from build123d import *

# Parameters (mm, degrees)
BOSS_EXTRUDE1_DEPTH = 5
SKETCH2_R           = 11.5
BOSS_EXTRUDE2_DEPTH = 35
BOSS_EXTRUDE3_DEPTH = 5
SKETCH4_R           = 0.75
CUT_EXTRUDE1_DEPTH  = 3
CUT_EXTRUDE2_REACH  = 47.957
SKETCH5_R           = 1
CHAMFER1_SIZE       = 1
CUT_EXTRUDE3_REACH  = 52.369
SKETCH6_R           = 8
FILLET2_R           = 5


with BuildPart() as part:
    # Sketch1 → Boss-Extrude1 (new body)
    with BuildSketch(Plane(origin=(0, 0, 0), x_dir=(1, 0, 0), z_dir=(0, 1, 0))):
        with BuildLine():
            Line((-14, 16), (14, 16))
            ThreePointArc((14, 16), (15.414213562, 15.414213562), (16, 14))
            Line((16, 14), (16, -14))
            ThreePointArc((16, -14), (15.414213562, -15.414213562), (14, -16))
            Line((14, -16), (-14, -16))
            ThreePointArc((-14, -16), (-15.414213562, -15.414213562), (-16, -14))
            Line((-16, -14), (-16, 14))
            ThreePointArc((-16, 14), (-15.414213562, 15.414213562), (-14, 16))
        make_face()
    extrude(amount=BOSS_EXTRUDE1_DEPTH)

    # Sketch2 → Boss-Extrude2 (add)
    with BuildSketch(Plane(origin=(0, 5, 0), x_dir=(1, 0, 0), z_dir=(0, 1, 0))):
        with Locations(Location((0, 0, 0), (0, 0, 270))):
            Circle(SKETCH2_R)
    extrude(amount=BOSS_EXTRUDE2_DEPTH)

    # Sketch3 → Boss-Extrude3 (add)
    with BuildSketch(Plane(origin=(0, 40, 0), x_dir=(1, 0, 0), z_dir=(0, 1, 0))):
        with BuildLine():
            Line((-14, 16), (14, 16))
            ThreePointArc((14, 16), (15.414213562, 15.414213562), (16, 14))
            Line((16, 14), (16, -14))
            ThreePointArc((16, -14), (15.414213562, -15.414213562), (14, -16))
            Line((14, -16), (-14, -16))
            ThreePointArc((-14, -16), (-15.414213562, -15.414213562), (-16, -14))
            Line((-16, -14), (-16, 14))
            ThreePointArc((-16, 14), (-15.414213562, 15.414213562), (-14, 16))
        make_face()
    extrude(amount=BOSS_EXTRUDE3_DEPTH)

    # Sketch4 → Cut-Extrude1 (cut)
    with BuildSketch(Plane.XZ):
        with Locations(Location((-13.651323601, 13.573265233, 0), (0, 0, 270))):
            Circle(SKETCH4_R)
        with Locations(Location((13.348541156, 13.658723546, 0), (0, 0, 270))):
            Circle(SKETCH4_R)
        with Locations(Location((13.43399947, -13.34114121, 0), (0, 0, 270))):
            Circle(SKETCH4_R)
        with Locations(Location((-13.565865287, -13.426599524, 0), (0, 0, 270))):
            Circle(SKETCH4_R)
    extrude(amount=-CUT_EXTRUDE1_DEPTH, mode=Mode.SUBTRACT)

    # Sketch5 → Cut-Extrude2 (cut, up to next)
    with BuildSketch(Plane.XZ.offset(-40), mode=Mode.PRIVATE) as cut_extrude2_sk1:
        with Locations(Location((-13.651323601, 13.573265233, 0), (0, 0, 270))):
            Circle(SKETCH5_R)
    cut_extrude2_tool1 = extrude(cut_extrude2_sk1.sketch, amount=-CUT_EXTRUDE2_REACH, mode=Mode.PRIVATE) & part.part
    # Sketch5 → Cut-Extrude2 (cut, up to next)
    with BuildSketch(Plane.XZ.offset(-40), mode=Mode.PRIVATE) as cut_extrude2_sk2:
        with Locations(Location((13.348541156, 13.658723546, 0), (0, 0, 270))):
            Circle(SKETCH5_R)
    cut_extrude2_tool2 = extrude(cut_extrude2_sk2.sketch, amount=-CUT_EXTRUDE2_REACH, mode=Mode.PRIVATE) & part.part
    # Sketch5 → Cut-Extrude2 (cut, up to next)
    with BuildSketch(Plane.XZ.offset(-40), mode=Mode.PRIVATE) as cut_extrude2_sk3:
        with Locations(Location((-13.565865287, -13.426599524, 0), (0, 0, 270))):
            Circle(SKETCH5_R)
    cut_extrude2_tool3 = extrude(cut_extrude2_sk3.sketch, amount=-CUT_EXTRUDE2_REACH, mode=Mode.PRIVATE) & part.part
    # Sketch5 → Cut-Extrude2 (cut, up to next)
    with BuildSketch(Plane.XZ.offset(-40), mode=Mode.PRIVATE) as cut_extrude2_sk4:
        with Locations(Location((13.43399947, -13.34114121, 0), (0, 0, 270))):
            Circle(SKETCH5_R)
    cut_extrude2_tool4 = extrude(cut_extrude2_sk4.sketch, amount=-CUT_EXTRUDE2_REACH, mode=Mode.PRIVATE) & part.part
    add(cut_extrude2_tool1.solids().sort_by_distance((-13.651324, 40, 13.573265))[0], mode=Mode.SUBTRACT)
    add(cut_extrude2_tool2.solids().sort_by_distance((13.348541, 40, 13.658724))[0], mode=Mode.SUBTRACT)
    add(cut_extrude2_tool3.solids().sort_by_distance((-13.565865, 40, -13.4266))[0], mode=Mode.SUBTRACT)
    add(cut_extrude2_tool4.solids().sort_by_distance((13.433999, 40, -13.341141))[0], mode=Mode.SUBTRACT)

    # Chamfer1
    chamfer1_edges = [part.edges().sort_by_distance(p)[0] for p in [
        (13.348541156, 40, 14.658723546),
        (-13.565865287, 40, -12.426599524),
        (13.43399947, 40, -12.34114121),
        (-13.651323601, 40, 14.573265233),
    ]]
    chamfer(chamfer1_edges, length=CHAMFER1_SIZE)

    # Sketch6 → Cut-Extrude3 (cut, up to next)
    with BuildSketch(Plane.XZ, mode=Mode.PRIVATE) as cut_extrude3_sk1:
        with Locations(Location((0, 0, 0), (0, 0, 270))):
            Circle(SKETCH6_R)
    cut_extrude3_tool1 = extrude(cut_extrude3_sk1.sketch, amount=-CUT_EXTRUDE3_REACH, mode=Mode.PRIVATE) & part.part
    add(cut_extrude3_tool1.solids().sort_by_distance((0, 0, 0))[0], mode=Mode.SUBTRACT)

    # Fillet2
    fillet2_edges = [part.edges().sort_by_distance(p)[0] for p in [
        (0, 5, -11.5),
        (0, 40, -11.5),
    ]]
    fillet(fillet2_edges, radius=FILLET2_R)


solid = part.part
The listing builds one solid part. Answer for the finished solid, in the listing's coordinates (mm). A direction names the side the tool comes from. Coordinates: 2 decimals unless noted, no trailing zeros. Loops run counter-clockwise (first coordinate to the right, second up) from the corner with the lowest first, then second, coordinate; pieces in that order, holes last.
1) Determine the mould class of faces 1 (the face through (-15.4, 42.46, 15.43)), 2 (the face through (-13.607, 42.972, 14.572)), 3 (the face through (11.4, 22.3, -1.5)) for opening direction Z: pulls with the +Z half, pulls with the -Z half, needs draft (parallel to the pull), parting line crosses it, or undercut.
2) Flat-ended cylindrical pins translate along their axes: pin 1 Ø12 at (y, z) = (31.5, -7) entering from +X; pin 2 Ø1.2 at (x, z) = (-13.65, 13.57) entering from +Y; pin 3 Ø8 at (y, z) = (25.5, -6.5) entering from -X (3 decimals). Find the tip coordinate at first contact, or state that the pin passes through.
3) A tool of negligible diameter and unlimited length cuts with its end or side. For faces 4 (the face through (12.547, 42.972, -13.803)), 5 (the face through (-13, 5, 12)), 6 (the face through (13, 3, -13)), from which of +Z, -Z, +X, -X, +Y, -Y can it reach the whole face along a straight path? Write none if from no direction.
4) Find the intervals of material crossed by L1, parallel to X at y = 28, z = 0; L2, parallel to Z at x = 2.5, y = 38; L3, parallel to Z at x = -6, y = 14.5, in increasing order.
5) Find section A-A on y = 27. Write down the section's boundary in (x, z).
Values:
1. face 1: pulls with the +Z half
1. face 2: undercut
1. face 3: parting line crosses it
2. pin 1: stops at x = 11.46
2. pin 2: stops at y = 5
2. pin 3: stops at x = -11.225
3. face 4: +Y
3. face 5: +Z, -X
3. face 6: -Y
4. L1: x = -11.5 to -8, 8 to 11.5
4. L2: z = -12.25 to -7.6, 7.6 to 12.25
4. L3: z = -9.81 to -5.29, 5.29 to 9.81
5. outline: circle Ø23 at (0, 0); hole circle Ø16 at (0, 0)
